```python
from build123d import *

# Parameters (mm, degrees)
SKETCH1_W           = 63.5
SKETCH1_H           = 139.7
SKETCH1_R           = 1.4224
SKETCH1_R_2         = 2.38125
BOSS_EXTRUDE1_DEPTH = 5.9944


with BuildPart() as part:
    # Sketch1 → Boss-Extrude1 (new body)
    with BuildSketch(Plane.XY):
        with Locations((31.75, 69.85)):
            Rectangle(SKETCH1_W, SKETCH1_H)
        with Locations((6.35, 133.35)):
            Circle(SKETCH1_R, mode=Mode.SUBTRACT)
        with Locations((57.15, 133.35)):
            Circle(SKETCH1_R, mode=Mode.SUBTRACT)
        with Locations((57.15, 6.35)):
            Circle(SKETCH1_R, mode=Mode.SUBTRACT)
        with Locations((6.35, 6.35)):
            Circle(SKETCH1_R, mode=Mode.SUBTRACT)
        with Locations((31.75, 44.8945)):
            Circle(SKETCH1_R_2, mode=Mode.SUBTRACT)
        Polygon((25.481826149, 104.411127028), (25.481826149, 113.369073478), (11.841725896, 99.728973225), (16.320699121, 95.25), align=None, mode=Mode.SUBTRACT)
        Polygon((25.481826149, 117.859201538), (25.481826149, 126.817147988), (11.841725896, 113.177047735), (16.320699121, 108.69807451), align=None, mode=Mode.SUBTRACT)
    extrude(amount=BOSS_EXTRUDE1_DEPTH)


solid = part.part
```
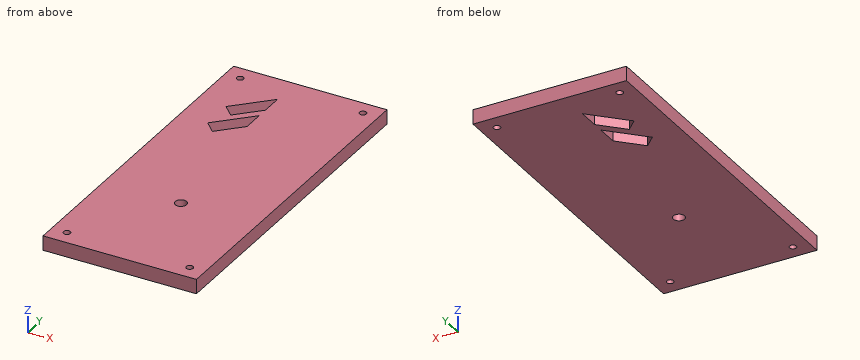
Geometry: final body of the model. Coordinates: model frame, mm. Coordinates: 2 decimals unless noted, no trailing zeros. Order: outer loops, then holes, each group sorted by start corner. A loop starts at its lowest first (then second) coordinate and runs counter-clockwise, first axis right, second up. Notation, with made-up numbers: M 82.5,-33 L 101.5,-33 A19 ccw 101.5,-29 Z; hole C -22.5,-34 d9. An arc over 180 degrees is marked long. Answer as CSV lines item,"result".
Q1. Section A-A on y = 6.35. Return the cut outline in (x, z), and give its area (3 significant figures).
Answers:
outline,"M 0,0 L 4.93,0 L 4.93,5.99 L 0,5.99 Z; M 7.77,0 L 55.73,0 L 55.73,5.99 L 7.77,5.99 Z; M 58.57,0 L 63.5,0 L 63.5,5.99 L 58.57,5.99 Z"
area,"347 mm^2"
Q2. Section C-C on z = 4.85. Return the cut outline in (x, y), and give its area (3 significant figures).
Answers:
outline,"M 0,0 L 63.5,0 L 63.5,139.7 L 0,139.7 Z; hole C 6.35,6.35 d2.84; hole C 6.35,133.35 d2.84; hole M 11.84,99.73 L 16.32,95.25 L 25.48,104.41 L 25.48,113.37 Z; hole M 11.84,113.18 L 16.32,108.7 L 25.48,117.86 L 25.48,126.82 Z; hole C 31.75,44.89 d4.76; hole C 57.15,6.35 d2.84; hole C 57.15,133.35 d2.84"
area,"8,620 mm^2"
Q3. Section D-D on x = 31. Return the cut outline in (y, z), and give its area (3 significant figures).
Answers:
outline,"M 0,0 L 42.63,0 L 42.63,5.99 L 0,5.99 Z; M 47.15,0 L 139.7,0 L 139.7,5.99 L 47.15,5.99 Z"
area,"810 mm^2"
Q4. Section B-B on x = 57.15. Return the cut outline in (y, z).
Answers:
outline,"M 0,0 L 4.93,0 L 4.93,5.99 L 0,5.99 Z; M 7.77,0 L 131.93,0 L 131.93,5.99 L 7.77,5.99 Z; M 134.77,0 L 139.7,0 L 139.7,5.99 L 134.77,5.99 Z"
Q5. Line query: probe 1 along Y at (x, z) = (6.35, 3); probe 2 along Y at (x, z) = (31.75, 3.6); probe 3 along Y at (x, z) = (18, 0.85). Output: solid intervals per line, ascending. Write a range as [from, to].
Answers:
probe 1,"y = [0, 4.93], [7.77, 131.93], [134.77, 139.7]"
probe 2,"y = [0, 42.51], [47.28, 139.7]"
probe 3,"y = [0, 96.93], [105.89, 110.38], [119.34, 139.7]"
